Drawing for the job (mm, zero at the part's lowest x, y, z). A direction names the side the tool comes from. Coordinates: 2 decimals unless noted, no trailing zeros. Write each loop counter-clockwise with the first axis right and the second up, starting at its lowest first coordinate (ties: lowest second). Pieces come first, ordered by that corner, then holes. Notation, with made-up numbers: (37, -33.5) -> (96, -33.5) arc R23 ccw to (96, -7.5) -> close; hole circle Ø5 at (-15.5, -31.75). An arc over 180 degrees is marked (long way). Write item = value, one per line. Start each with the question number.
Q1. Band-saw the part on A-A, the plane z = 8.5. List the corners of the cut face in (x, y).
Q2. Probe line 1 (Y direction, x = 35.75, z = 22.65); line 2 (X direction, y = 41, z = 9.75); line 3 (Z direction, x = 47, y = 62.4). List the from-to ranges inside material, lowest first.
Q3. Band-saw the part on C-C, the plane y = 4.75. List the corners of the cut face in (x, z).
Q4. Tool access for the marked faces 1, 2, 3 and 4: list every direction of +Z, -Z, +X, -X, +Y, -Y with a clear straight run to the whole face (end or side of a thin tool).
Q5. Band-saw the part on B-B, the plane x = 35.75. List the corners of the cut face in (y, z), plus the area to 3 significant figures.
Q6. Pin check, flat tips, straight feed: P1, Ø3, axis at x = 56.5, y = 27, coming from the -Z side; P2, Ø10, axis at x = 39, z = 13.5, coming from the -Y side; P3, Ø1.5, axis at x = 36, z = 7.5, coming from the +Y side. Stop position of each tip, or through.
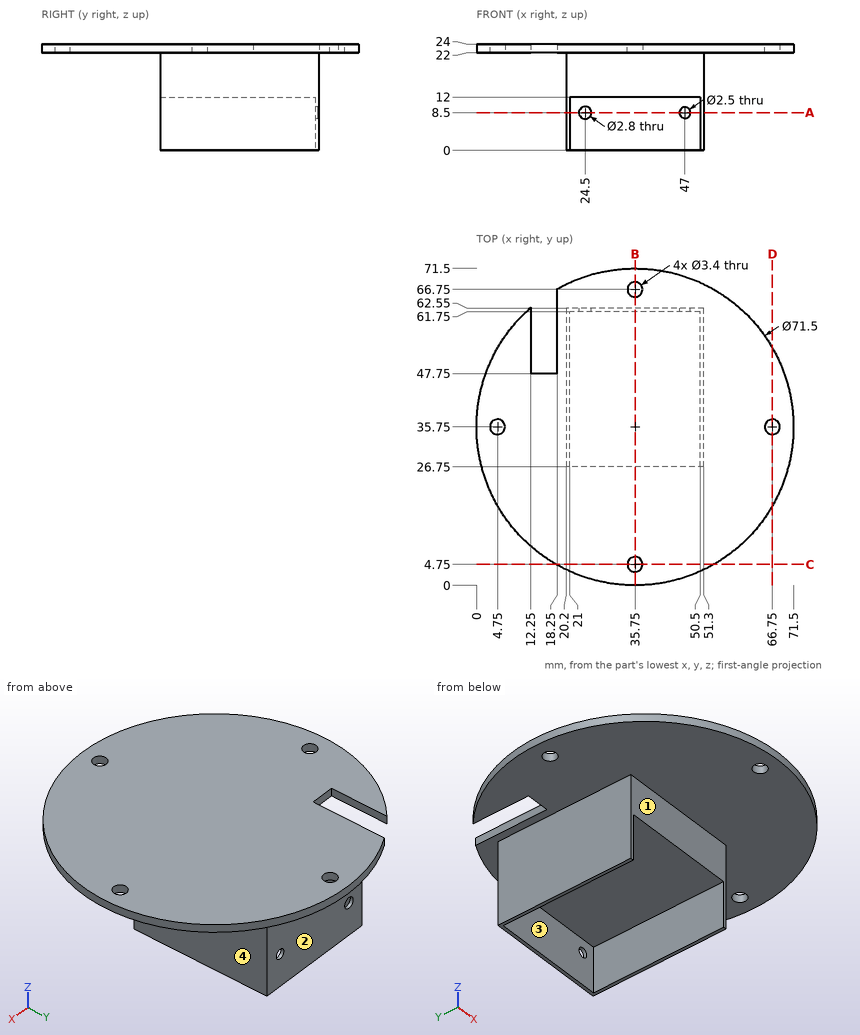
Ans:
q1.outline = (20.2, 26.75) -> (21, 26.75) -> (21, 61.75) -> (23.1, 61.75) -> (23.1, 62.55) -> (20.2, 62.55) -> close; (25.9, 61.75) -> (45.75, 61.75) -> (45.75, 62.55) -> (25.9, 62.55) -> close; (48.25, 61.75) -> (50.5, 61.75) -> (50.5, 26.75) -> (51.3, 26.75) -> (51.3, 62.55) -> (48.25, 62.55) -> close
q2.line_1 = 0 to 3.05, 6.45 to 65.05, 68.45 to 71.5
q2.line_2 = 20.2 to 21, 50.5 to 51.3
q2.line_3 = 0 to 7.25, 9.75 to 24
q3.outline = (17.94, 22) -> (34.05, 22) -> (34.05, 24) -> (17.94, 24) -> close; (37.45, 22) -> (53.56, 22) -> (53.56, 24) -> (37.45, 24) -> close
q4.face_1 = -Z, +X, -X, -Y
q4.face_2 = -Z, +X, -X, +Y
q4.face_3 = -Z, -Y
q4.face_4 = -Z, +X, +Y, -Y
q5.outline = (0, 22) -> (3.05, 22) -> (3.05, 24) -> (0, 24) -> close; (6.45, 22) -> (26.75, 22) -> (26.75, 12) -> (61.75, 12) -> (61.75, 0) -> (62.55, 0) -> (62.55, 22) -> (65.05, 22) -> (65.05, 24) -> (6.45, 24) -> close; (68.45, 22) -> (71.5, 22) -> (71.5, 24) -> (68.45, 24) -> close
q5.area = 497 mm2
q6.P1 = 22
q6.P2 = 26.75
q6.P3 = 62.55
